Can you work these out from the model? Positions are in its coordinate system, mm. A direction names the side the tool comes from. Round coordinates to 2 decimals unless told otherwise and drop trailing zeros. Loops run counter-clockwise (first coordinate to the right, second up) from the corner with the lowest first, then second, coordinate; pieces in that order, holes last.
(1) I want a section at A-A on z = -4.5. Write out the boundary of the cut face in (x, y).
(2) Will these pins go through, and if not, where does the flat tip stop? pin 1 Ø1 at (y, z) = (8, -12) entering from +X; pin 2 Ø1 at (y, z) = (11.5, -16) entering from +X.
(3) I want a section at B-B on z = -13.5. Write out the boundary of the cut face in (x, y).
(4) If I drill on line 1 along X through (y, z) = (10.5, -6); line 2 along X through (y, z) = (14.25, -12); line 3 along X through (y, z) = (12.5, -2), over which ranges is the centre line in solid material (lowest first)?
(5) I want a section at C-C on y = 8.75. Write out the boundary of the cut face in (x, z), plus the area to 3 significant figures.
(6) Which directions (+Z, -Z, +X, -X, +Y, -Y) give clear straight access to the entire face, cutting with the end or side of a thin tool? Please do faces 4 (the face through (-18, 7, -8)), 5 (the face through (-4, 15, -9)), 6 (the face through (1.9, 7, -3)).
(7) I want a section at D-D on x = -12. Write out the boundary of the cut face in (y, z).
(8) Thinking about a two-plate mould opening in X: for faces 1 (the face through (1, 7, 0)), 2 (the face through (-12, 7, -25)), 3 (the face through (1, 7, 6)), which applies, released by +X, released by -X, zero draft, split by the parting line, or undercut?
Autodesk Inventor part; units mm, degrees
ref_plane "YZ Plane" through (0, 0, 0) normal (1, 0, 0) x (0, 1, 0)
ref_plane "XZ Plane" through (0, 0, 0) normal (0, 1, 0) x (-1, 0, 0)
ref_plane "XY Plane" through (0, 0, 0) normal (0, 0, 1) x (1, 0, 0)
sketch "Sketch1" plane through (0, 0, 0) normal (0, 1, 0) x (-1, 0, 0)
  line L0 (0, 0) -> (-1.9, 0)
  line L1 (-1.9, 0) -> (-1.9, -7)
  line L2 (-4.9, -10) -> (-4.9, -10)
  line L3 (-7.9, -7) -> (-7.9, 3)
  line L4 (-4.9, 6) -> (3, 6)
  line L5 (0, 0) -> (0, -13)
  line L6 (12, -25) -> (12, -25)
  line L7 (24, -13) -> (24, -4)
  line L8 (21, -1) -> (21, -1)
  line L9 (18, -4) -> (18, -13)
  line L10 (12, -19) -> (12, -19)
  line L11 (6, -13) -> (6, 3)
  arc A0 (6, -13) -> (12, -19) centre (12, -13) ccw
  arc A1 (12, -19) -> (18, -13) centre (12, -13) ccw
  arc A2 (0, -13) -> (12, -25) centre (12, -13) ccw
  arc A3 (12, -25) -> (24, -13) centre (12, -13) ccw
  arc A4 (-4.9, 6) -> (-7.9, 3) centre (-4.9, 3) ccw
  arc A5 (6, 3) -> (3, 6) centre (3, 3) ccw
  arc A6 (-4.9, -10) -> (-1.9, -7) centre (-4.9, -7) ccw
  arc A7 (-7.9, -7) -> (-4.9, -10) centre (-4.9, -7) ccw
  arc A8 (24, -4) -> (21, -1) centre (21, -4) ccw
  arc A9 (21, -1) -> (18, -4) centre (21, -4) ccw
  point P0 (-1.9, -10)
  point P1 (-7.9, -10)
  point P2 (-7.9, 6)
  point P3 (6, 6)
  point P4 (0, -25)
  point P5 (24, -25)
  point P6 (24, -1)
  point P7 (18, -1)
  point P8 (18, -19)
  point P9 (6, -19)
  dimension "d0" = 1.9
  dimension "d1" = 10
  dimension "d2" = 6
  dimension "d3" = 16
  dimension "d4" = 6
  dimension "d5" = 25
  dimension "d6" = 24
  dimension "d7" = 24
  dimension "d8" = 6
  dimension "d9" = 18
  dimension "d10" = 12
  dimension "d11" = 6
  dimension "d12" = 12
  dimension "d13" = 3
extrude "Extrusion1" add sketch "Sketch1" along normal blind 15
properties part number "Percha"
Filled sheet:
1. outline: (-24, 0) - (-18, 0) - (-18, 15) - (-24, 15) - close; (-6, 0) - (0, 0) - (0, 15) - (-6, 15) - close; (1.9, 0) - (7.9, 0) - (7.9, 15) - (1.9, 15) - close
2. pin 1: stops at x = 0
2. pin 2: stops at x = -0.26
3. outline: (-23.99, 0) - (-17.98, 0) - (-17.98, 15) - (-23.99, 15) - close; (-6.02, 0) - (-0.01, 0) - (-0.01, 15) - (-6.02, 15) - close
4. line 1: x = -24 to -18, -6 to 0, 1.9 to 7.9
4. line 2: x = -24 to -18, -6 to 0
4. line 3: x = -23.24 to -18.76, -6 to 0, 1.9 to 7.9
5. outline: (-24, -13) arc R12 ccw to (0, -13) - (0, 0) - (1.9, 0) - (1.9, -7) arc R3 ccw to (7.9, -7) - (7.9, 3) arc R3 ccw to (4.9, 6) - (-3, 6) arc R3 ccw to (-6, 3) - (-6, -13) arc R6 cw to (-18, -13) - (-18, -4) arc R3 ccw to (-24, -4) - close
5. area: 451 mm2
6. face 4: +Z, +Y, -Y
6. face 5: +Z, -Z, +X, -X, +Y
6. face 6: -Z, +Y, -Y
7. outline: (0, -25) - (15, -25) - (15, -19) - (0, -19) - close
8. face 1: undercut
8. face 2: split by the parting line
8. face 3: zero draft
